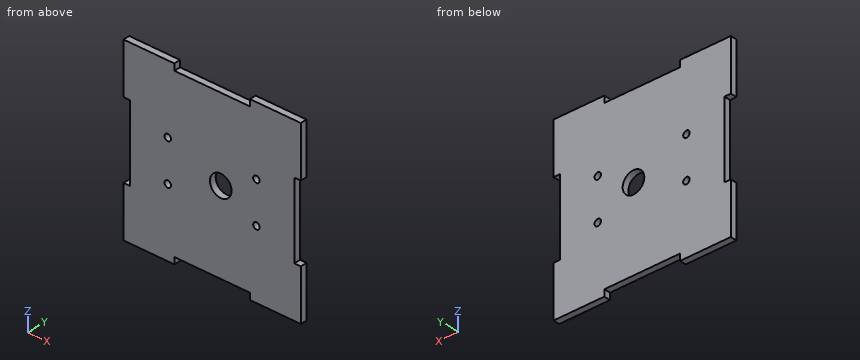
from build123d import *

# Parameters (mm, degrees)
BOSS_EXTRUDE1_DEPTH = 3
SKETCH2_R           = 5
SKETCH2_R_2         = 1.5
CUT_EXTRUDE1_DEPTH  = 3


with BuildPart() as part:
    # Sketch1 → Boss-Extrude1 (new body)
    with BuildSketch(Plane(origin=(0, 0, 0), x_dir=(1, 0, 0), z_dir=(0, 1, 0))):
        Polygon((-41, -41), (-17.5, -41), (-17.5, -38), (17.5, -38), (17.5, -41), (41, -41), (41, -17.5), (38, -17.5), (38, 17.5), (41, 17.5), (41, 41), (17.5, 41), (17.5, 38), (-17.5, 38), (-17.5, 41), (-41, 41), (-41, 17.5), (-38, 17.5), (-38, -17.5), (-41, -17.5), align=None)
    extrude(amount=BOSS_EXTRUDE1_DEPTH)

    # Sketch2 → Cut-Extrude1 (cut)
    with BuildSketch(Plane(origin=(0, 3, 0), x_dir=(1, 0, 0), z_dir=(0, 1, 0))):
        with Locations((4, 0)):
            Circle(SKETCH2_R)
        with Locations((-20.5, 9.5)):
            Circle(SKETCH2_R_2)
        with Locations((-20.5, -9.5)):
            Circle(SKETCH2_R_2)
        with Locations((20.5, -9.5)):
            Circle(SKETCH2_R_2)
        with Locations((20.5, 9.5)):
            Circle(SKETCH2_R_2)
    extrude(amount=-CUT_EXTRUDE1_DEPTH, mode=Mode.SUBTRACT)


solid = part.part
Build history of the part. All positions in model axes, mm. Coordinates: 2 decimals unless noted, no trailing zeros. Write each loop counter-clockwise with the first axis right and the second up, starting at its lowest first coordinate (ties: lowest second). Pieces come first, ordered by that corner, then holes.
(1) Drill centre lines: line 1 (Z direction, x = -20.5, y = 0.9); line 2 (X direction, y = 1.9, z = 9.5); line 3 (X direction, y = 1.3, z = -6). Where is each one in solid material? Low to high.
(2) Cut at A-A on z = 0. List the corners of the cut face in (x, y), and give its area (3 significant figures).
(3) Pin check, flat tips, straight feed: pin 1 Ø1.5 at (y, z) = (1.5, -9.5) entering from +X; pin 2 Ø2.5 at (x, z) = (-20.5, 9.5) entering from -Y; pin 3 Ø8 at (x, z) = (-1, 28.5) entering from -Y; pin 4 Ø1.5 at (x, y) = (5, 1) entering from +Z. Stop position of each tip, or through.
(4) Cut at D-D on y = 1.55. List the corners of the cut face in (x, z), and give its area (3 significant figures).
(5) Cut at C-C on z = -9.5. List the corners of the cut face in (x, y).
(6) Cut at B-B on x = 20.5. List the corners of the cut face in (y, z), and give its area (3 significant figures).
Working result:
1. line 1: z = -41 to -11, -8 to 8, 11 to 41
1. line 2: x = -38 to -22, -19 to 19, 22 to 38
1. line 3: x = -38 to 38
2. outline: (-38, 0) - (-1, 0) - (-1, 3) - (-38, 3) - close; (9, 0) - (38, 0) - (38, 3) - (9, 3) - close
2. area: 198 mm2
3. pin 1: stops at x = 38
3. pin 2: passes through
3. pin 3: stops at y = 0
3. pin 4: stops at z = 38
4. outline: (-41, -41) - (-17.5, -41) - (-17.5, -38) - (17.5, -38) - (17.5, -41) - (41, -41) - (41, -17.5) - (38, -17.5) - (38, 17.5) - (41, 17.5) - (41, 41) - (17.5, 41) - (17.5, 38) - (-17.5, 38) - (-17.5, 41) - (-41, 41) - (-41, 17.5) - (-38, 17.5) - (-38, -17.5) - (-41, -17.5) - close; hole circle Ø3 at (-20.5, -9.5); hole circle Ø3 at (-20.5, 9.5); hole circle Ø10 at (4, 0); hole circle Ø3 at (20.5, -9.5); hole circle Ø3 at (20.5, 9.5)
4. area: 6,200 mm2
5. outline: (-38, 0) - (-22, 0) - (-22, 3) - (-38, 3) - close; (-19, 0) - (19, 0) - (19, 3) - (-19, 3) - close; (22, 0) - (38, 0) - (38, 3) - (22, 3) - close
6. outline: (0, -41) - (3, -41) - (3, -11) - (0, -11) - close; (0, -8) - (3, -8) - (3, 8) - (0, 8) - close; (0, 11) - (3, 11) - (3, 41) - (0, 41) - close
6. area: 228 mm2
